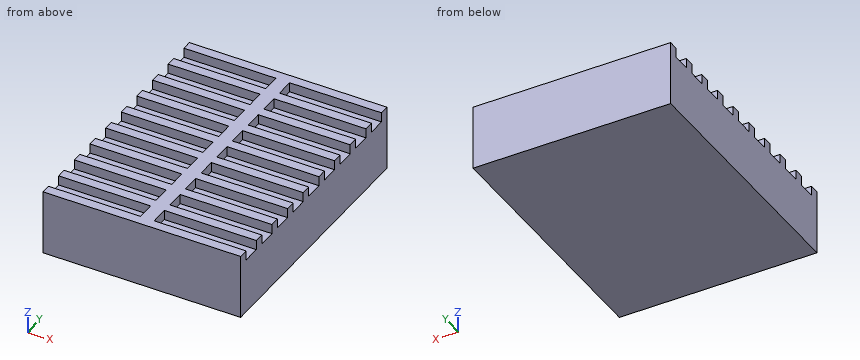
from build123d import *

# Parameters (mm, degrees)
SKETCH_1_W      = 14.3
SKETCH_1_H      = 18.7
EXTRUDE_1_DEPTH = 4
SKETCH_2_W      = 0.7
SKETCH_2_H      = 0.7
EXTRUDE_2_DEPTH = 14.3
SKETCH_3_W      = 1
SKETCH_3_H      = 18.7
EXTRUDE_4_DEPTH = 0.7


with BuildPart() as part:
    # 草图1 → 凸台-拉伸1 (new body)
    with BuildSketch(Plane.XY):
        with Locations((7.15, -9.35)):
            Rectangle(SKETCH_1_W, SKETCH_1_H)
    extrude(amount=EXTRUDE_1_DEPTH)

    # 草图2 → 凸台-拉伸2 (add)
    with BuildSketch(Plane(origin=(14.3, 0, 0), x_dir=(0, 0, -1), z_dir=(1, 0, 0))):
        with Locations((-4.35, -2.35)):
            Rectangle(SKETCH_2_W, SKETCH_2_H)
        with Locations((-4.35, -0.35)):
            Rectangle(SKETCH_2_W, SKETCH_2_H)
        with Locations((-4.35, -4.35)):
            Rectangle(SKETCH_2_W, SKETCH_2_H)
        with Locations((-4.35, -6.35)):
            Rectangle(SKETCH_2_W, SKETCH_2_H)
        with Locations((-4.35, -8.35)):
            Rectangle(SKETCH_2_W, SKETCH_2_H)
        with Locations((-4.35, -10.35)):
            Rectangle(SKETCH_2_W, SKETCH_2_H)
        with Locations((-4.35, -12.35)):
            Rectangle(SKETCH_2_W, SKETCH_2_H)
        with Locations((-4.35, -14.35)):
            Rectangle(SKETCH_2_W, SKETCH_2_H)
        with Locations((-4.35, -16.35)):
            Rectangle(SKETCH_2_W, SKETCH_2_H)
        with Locations((-4.35, -18.35)):
            Rectangle(SKETCH_2_W, SKETCH_2_H)
    extrude(amount=-EXTRUDE_2_DEPTH)

    # 草图3 → 凸台-拉伸4 (add)
    with BuildSketch(Plane.XY.offset(4)):
        with Locations((7.15, -9.35)):
            Rectangle(SKETCH_3_W, SKETCH_3_H)
    extrude(amount=EXTRUDE_4_DEPTH)


solid = part.part
Build history of the part. All positions in model axes, mm. Round coordinates to 2 decimals unless told otherwise and drop trailing zeros. Loops run counter-clockwise (first coordinate to the right, second up) from the corner with the lowest first, then second, coordinate; pieces in that order, holes last. Notation, with made-up numbers: (20, 12) -> (55, 12) arc R18 ccw to (55, 43) -> close; hole circle Ø4 at (86.25, -22.5). An arc over 180 degrees is marked (long way). One line per item, written item: value. Start each with the question number.
Q1. Probe line 1 along Z through (x, y) = (10, -1.5); line 2 along X through (y, z) = (-5, 4.45). List the from-to ranges inside material, lowest first.
Q2. Cut at A-A on y = -11.75. List the corners of the cut face in (x, z), plus the area to 3 significant figures.
Q3. Drop flat-ended pins along their axis: pin 1 Ø0.8 at (y, z) = (-15.5, 4.5) entering from +X; pin 2 Ø0.7 at (x, y) = (11, -5.5) entering from +Z. Give the stop position or say it passes through.
Computed:
1. line 1: 0 to 4
1. line 2: 6.65 to 7.65
2. outline: (0, 0) -> (14.3, 0) -> (14.3, 4) -> (7.65, 4) -> (7.65, 4.7) -> (6.65, 4.7) -> (6.65, 4) -> (0, 4) -> close
2. area: 57.9 mm²
3. pin 1: x = 7.65
3. pin 2: z = 4
